Verification items for the finished model (mm, model axes). A direction names the side the tool comes from. Round coordinates to 2 decimals unless told otherwise and drop trailing zeros. Order: outer loops, then holes, each group sorted by start corner. A loop starts at its lowest first (then second) coordinate and runs counter-clockwise, first axis right, second up. Notation, with made-up numbers: (83.25, 61) -> (123.25, 61) arc R10 cw to (123.25, 80) -> close; hole circle Ø11 at (84, 27.5). An arc over 180 degrees is marked (long way). Return JSON: item names as keys, results as strings. Group by question number.
Item 1: Sectioned sample at C-C on x = 139.7. Record the cut outline in (y, z), plus the area to 3 significant figures.
Item 2: Access from +Z, -Z, +X, -X, +Y, -Y to the whole of each face (thin tool, end or side, straight path). Record for faces 4 (the flat face through (1, 3, 3.429)), 5 (the flat face through (152.4, 3, 0)).
Item 3: Scan lines: probe 1 along X at (y, z) = (3, 19.05); probe 2 along Z at (x, y) = (-139.7, 4.75); probe 3 along Z at (x, y) = (27, 4). Record each from-to range of solid material in increasing order. Write a range as from..to.
Item 4: Depth check by flat-ended pin: pin 1 Ø6 at (x, z) = (-139.7, 19.05) entering from -Y; pin 2 Ø4.5 at (x, z) = (-139.7, -19.05) entering from +Y. Enter the tip coordinate at first touch or a pass-through.
Item 5: Sectioned sample at A-A on x = 0. Record the cut outline in (y, z), plus the area to 3 significant figures.
Item 6: Sectioned sample at D-D on y = 1.75. Record the cut outline in (x, z).
Item 7: Sectioned sample at B-B on z = 19.05. Record the cut outline in (x, y).
Item 8: Draft check along Z on faces 1 (the flat face through (-152.4, 3, 0)), 2 (the cylindrical face through (103.43, 3.13, -0.08)), 3 (the flat face through (-2, 3, -31.75)). Enter one of: pulls with the +Z half, pulls with the -Z half, needs draft (parallel to the pull), parting line crosses it, or undercut.
```python
from build123d import *

# Parameters (mm, degrees)
SKETCH1_W           = 304.8
SKETCH1_H           = 63.5
SKETCH1_R           = 2.5796875
BOSS_EXTRUDE1_DEPTH = 6.35


with BuildPart() as part:
    # Sketch1 → Boss-Extrude1 (new body)
    with BuildSketch(Plane(origin=(0, 0, 0), x_dir=(1, 0, 0), z_dir=(0, 1, 0))):
        Rectangle(SKETCH1_W, SKETCH1_H)
        with Locations(Location((-139.7, 19.05, 0), (0, 0, 270))):
            Circle(SKETCH1_R, mode=Mode.SUBTRACT)
        with Locations(Location((139.7, 19.05, 0), (0, 0, 90))):
            Circle(SKETCH1_R, mode=Mode.SUBTRACT)
        with Locations(Location((139.7, -19.05, 0), (0, 0, 270))):
            Circle(SKETCH1_R, mode=Mode.SUBTRACT)
        with Locations(Location((-139.7, -19.05, 0), (0, 0, 90))):
            Circle(SKETCH1_R, mode=Mode.SUBTRACT)
        with BuildLine():
            Line((-100, 3.429), (100, 3.429))
            ThreePointArc((100, 3.429), (103.429, 0), (100, -3.429))
            Line((100, -3.429), (-100, -3.429))
            ThreePointArc((-100, -3.429), (-103.429, 0), (-100, 3.429))
        make_face(mode=Mode.SUBTRACT)
    extrude(amount=BOSS_EXTRUDE1_DEPTH)


solid = part.part
```
Recorded:
{
 "1": {"outline": "(0, -31.75) -> (6.35, -31.75) -> (6.35, -21.63) -> (0, -21.63) -> close; (0, -16.47) -> (6.35, -16.47) -> (6.35, 16.47) -> (0, 16.47) -> close; (0, 21.63) -> (6.35, 21.63) -> (6.35, 31.75) -> (0, 31.75) -> close", "area": "338 mm²"},
 "2": {"face 4": "+Y, -Y", "face 5": "+Z, -Z, +X, +Y, -Y"},
 "3": {"probe 1": "-152.4..-142.28, -137.12..137.12, 142.28..152.4", "probe 2": "-31.75..-21.63, -16.47..16.47, 21.63..31.75", "probe 3": "-31.75..-3.43, 3.43..31.75"},
 "4": {"pin 1": "y = 0", "pin 2": "through"},
 "5": {"outline": "(0, -31.75) -> (6.35, -31.75) -> (6.35, -3.43) -> (0, -3.43) -> close; (0, 3.43) -> (6.35, 3.43) -> (6.35, 31.75) -> (0, 31.75) -> close", "area": "360 mm²"},
 "6": {"outline": "(-152.4, -31.75) -> (152.4, -31.75) -> (152.4, 31.75) -> (-152.4, 31.75) -> close; hole circle Ø5.16 at (-139.7, -19.05); hole circle Ø5.16 at (-139.7, 19.05); hole (-100, -3.43) -> (100, -3.43) arc R3.43 ccw to (100, 3.43) -> (-100, 3.43) arc R3.43 ccw to start; hole circle Ø5.16 at (139.7, -19.05); hole circle Ø5.16 at (139.7, 19.05)"},
 "7": {"outline": "(-152.4, 0) -> (-142.28, 0) -> (-142.28, 6.35) -> (-152.4, 6.35) -> close; (-137.12, 0) -> (137.12, 0) -> (137.12, 6.35) -> (-137.12, 6.35) -> close; (142.28, 0) -> (152.4, 0) -> (152.4, 6.35) -> (142.28, 6.35) -> close"},
 "8": {"face 1": "needs draft", "face 2": "undercut", "face 3": "pulls with the -Z half"}
}
